from build123d import *

# Parameters (mm, degrees)
F0_R        = 14
F1_DEPTH    = 8.05
F2_T1_DEPTH = 8.05
F3_SIZE     = 0.99999


# Not quite as in the source:
# - a fillet or chamfer that OpenCascade refuses, or shapes differently, is made with other operations: its cross-section is extruded or revolved along the edge and cut away or added
# - a fillet or chamfer is up to 0.001 mm smaller than in the source, because OpenCascade refuses the exact size


with BuildPart() as f1:
    # F0 (on Top) → F1 (new body)
    with BuildSketch(Plane.XY):
        with BuildLine():
            ThreePointArc((-18.9934809997, -0.4976741041), (-16.4544826719, -9.5), (-9.9277389168, -16.2))
            ThreePointArc((-9.9277389168, -16.2), (0, -47), (9.9277389168, -16.2))
            ThreePointArc((9.9277389168, -16.2), (16.4544826719, -9.5), (18.9934809997, -0.4976741041))
            ThreePointArc((18.9934809997, -0.4976741041), (40.7031939779, 23.5), (9.0657420829, 16.6976741041))
            ThreePointArc((9.0657420829, 16.6976741041), (0, 19), (-9.0657420829, 16.6976741041))
            ThreePointArc((-9.0657420829, 16.6976741041), (-40.7031939779, 23.5), (-18.9934809997, -0.4976741041))
        make_face()
        with BuildLine():
            ThreePointArc((5.9, -17.3039376183), (6.3427828622, -17.5192506009), (6.7777208559, -17.75))
            ThreePointArc((6.7777208559, -17.75), (12.0600184905, -22.8897289778), (14, -30))
            ThreePointArc((14, -30), (-7.5299402388, -41.8025420991), (-5.9, -17.3039376183))
            ThreePointArc((-5.9, -17.3039376183), (0, -16), (5.9, -17.3039376183))
        make_face(mode=Mode.SUBTRACT)
        with BuildLine():
            ThreePointArc((-17.9356495629, 3.5424189268), (-38.4031526988, 21.4563311676), (-11.9807621135, 15))
            ThreePointArc((-11.9807621135, 15), (-11.9944907071, 14.3801515137), (-12.0356495629, 13.7615186915))
            ThreePointArc((-12.0356495629, 13.7615186915), (-13.8564064606, 8), (-17.9356495629, 3.5424189268))
        make_face(mode=Mode.SUBTRACT)
        Circle(F0_R, mode=Mode.SUBTRACT)
        with BuildLine():
            ThreePointArc((11.9830904892, 14.7446784409), (25.8530960258, 28.999417894), (39.9807621135, 15))
            ThreePointArc((39.9807621135, 15), (32.4370932811, 2.5776094147), (17.9356495629, 3.5424189268))
            ThreePointArc((17.9356495629, 3.5424189268), (13.8564064606, 8), (12.0356495629, 13.7615186915))
            ThreePointArc((12.0356495629, 13.7615186915), (12.0007246446, 14.2526363898), (11.9830904892, 14.7446784409))
        make_face(mode=Mode.SUBTRACT)
    extrude(amount=F1_DEPTH)

    # F2: fillet of radius 20 on 6 edges, made by hand

    # F2_s2 → F2_t1 (join)
    with BuildSketch(Plane.XY):
        with BuildLine():
            ThreePointArc((-15.8833011878, -10.4269239653), (-21.5600561339, -4.7274127209), (-29.0232123622, -1.725534266))
            ThreePointArc((-29.0232123622, -1.725534266), (-23.9150097608, -1.8740234448), (-18.9934809997, -0.4976741041))
            ThreePointArc((-18.9934809997, -0.4976741041), (-18.1313260585, -5.6793499065), (-15.8833011878, -10.4269239653))
        make_face()
        with BuildLine():
            ThreePointArc((-16.9716316312, -8.5418803419), (-14.8740875774, -16.3078499586), (-16.0059626906, -24.2720720721))
            ThreePointArc((-16.0059626906, -24.2720720721), (-13.5804567909, -19.7739942621), (-9.9277389168, -16.2))
            ThreePointArc((-9.9277389168, -16.2), (-13.9841243252, -12.8625140177), (-16.9716316312, -8.5418803419))
        make_face()
        with BuildLine():
            ThreePointArc((-1.0883304434, 18.9688043072), (6.6859685565, 21.0352626795), (13.0172496716, 25.9976063381))
            ThreePointArc((13.0172496716, 25.9976063381), (10.3345529699, 21.648017707), (9.0657420829, 16.6976741041))
            ThreePointArc((9.0657420829, 16.6976741041), (4.1472017333, 18.5418639242), (-1.0883304434, 18.9688043072))
        make_face()
        with BuildLine():
            ThreePointArc((1.0883304434, 18.9688043072), (-6.6859685565, 21.0352626795), (-13.0172496716, 25.9976063381))
            ThreePointArc((-13.0172496716, 25.9976063381), (-10.3345529699, 21.648017707), (-9.0657420829, 16.6976741041))
            ThreePointArc((-9.0657420829, 16.6976741041), (-4.1472017333, 18.5418639242), (1.0883304434, 18.9688043072))
        make_face()
        with BuildLine():
            ThreePointArc((29.0232123622, -1.725534266), (21.5600561339, -4.7274127209), (15.8833011878, -10.4269239653))
            ThreePointArc((15.8833011878, -10.4269239653), (18.1313260585, -5.6793499065), (18.9934809997, -0.4976741041))
            ThreePointArc((18.9934809997, -0.4976741041), (23.9150097608, -1.8740234448), (29.0232123622, -1.725534266))
        make_face()
        with BuildLine():
            ThreePointArc((16.9716316312, -8.5418803419), (14.8740875774, -16.3078499586), (16.0059626906, -24.2720720721))
            ThreePointArc((16.0059626906, -24.2720720721), (13.5804567909, -19.7739942621), (9.9277389168, -16.2))
            ThreePointArc((9.9277389168, -16.2), (13.9841243252, -12.8625140177), (16.9716316312, -8.5418803419))
        make_face()
    extrude(amount=F2_T1_DEPTH)

    # F3 (size 1 in the source; OpenCascade refuses exactly that, so slightly less here)
    f3_edges = [f1.edges().sort_by_distance(p)[0] for p in [
        (0, -47, 8.05),
        (14.848068, -16.8534, 8.05),
        (22.019507, -4.432104, 8.05),
        (40.703194, 23.5, 8.05),
        (7.171439, 21.285504, 8.05),
        (-7.171439, 21.285504, 8.05),
        (-40.703194, 23.5, 8.05),
        (-22.019507, -4.432104, 8.05),
        (-14.848068, -16.8534, 8.05),
        (5.9, -42.696062, 8.05),
        (-39.980762, 15, 8.05),
        (-14, 0, 8.05),
        (11.980762, 15, 8.05),
    ]]
    chamfer(f3_edges, length=F3_SIZE)


solid = f1.part
CAD build for the part. Positions are in the model's coordinates, mm. A direction names the side the tool comes from. Round coordinates to 2 decimals unless told otherwise and drop trailing zeros. Order: outer loops, then holes, each group sorted by start corner. A loop starts at its lowest first (then second) coordinate and runs counter-clockwise, first axis right, second up. Notation, with made-up numbers: (76.5, 73) - (122.5, 73) arc R18 cw to (122.5, 106) - close; hole circle Ø3 at (35, 88.5). An arc over 180 degrees is marked (long way). Return JSON: item names as keys, results as strings.
(1) Cut at A-A (z = 3.5). Give the cut face in (x, y).
Answer key:
{"outline": "(-29.02, -1.73) arc R20 cw to (-16.51, -9.53) arc R20 cw to (-16.01, -24.27) arc R17 ccw (long way) to (16.01, -24.27) arc R20 cw to (16.51, -9.53) arc R20 cw to (29.02, -1.73) arc R17 ccw (long way) to (13.02, 26) arc R20 cw to (0, 19.06) arc R20 cw to (-13.02, 26) arc R17 ccw (long way) to start; hole circle Ø28 at (-25.98, 15); hole circle Ø28 at (0, -30); hole circle Ø28 at (0, 0); hole circle Ø28 at (25.98, 15)"}
(2) Tool access for faces 1 (the face through (0.2, 15.5, 8.05)), 2 (the face through (-7.078, 21.236, 3.476)): list every direction of +Z, -Z, +X, -X, +Y, -Y with a clear straight run to the whole face (end or side of a thin tool).
Answer key:
{"face 1": "+Z, +X, -X, +Y, -Y", "face 2": "+Z, -Z, +Y"}
(3) Pull direction Y, two halves, no side cores. Call faces 3 (the face through (7.078, 21.236, 3.476)), 4 (the face through (0, -47, 3)), 5 (the face through (-14.85, -16.75, 3.48)), 6 (the face through (-40.47, 23.89, 3.48)): +Y half, -Y half, draft (parallel to the pull), parting line (faces both ways), or undercut.
Answer key:
{"face 3": "+Y half", "face 4": "undercut", "face 5": "undercut", "face 6": "parting line"}
(4) Wall check: probe 1 along X at (y, z) = (15.5, 4.25); probe 2 along Y at (x, z) = (-0.5, 1.25); probe 3 along X at (y, z) = (-30, 4). Give the ranges that are in metal, low to high. Write a range as from..to.
Answer key:
{"probe 1": "x = -42.97..-39.97, -11.99..11.99, 39.97..42.97", "probe 2": "y = -46.99..-43.99, -16.01..-13.99, 13.99..19.12", "probe 3": "x = -17..-14, 14..17"}
(5) Pin check, flat tips, straight feed: pin 1 Ø2 at (x, z) = (-25, 3) entering from -Y; pin 2 Ø25 at (x, y) = (0, 0) entering from -Z; pin 3 Ø1 at (y, z) = (4, 7) entering from -X. Stop position of each tip, or through.
Answer key:
{"pin 1": "stops at y = -3.35", "pin 2": "passes through", "pin 3": "stops at x = -39.35"}
(6) Cut at B-B (x = -3.5). State how many separate pieces and enclosed holes the cut face has, then the cut area to 3 significant figures.
Answer key:
{"separate pieces": "3", "enclosed holes": "0", "area": "95.0 mm^2"}
